The model under review builds one solid part; all positions refer to its coordinate system, in mm. Face numbers are marked on the shaded views. Coordinates: 2 decimals unless noted, no trailing zeros. Write each loop counter-clockwise with the first axis right and the second up, starting at its lowest first coordinate (ties: lowest second). Pieces come first, ordered by that corner, then holes. Notation, with made-up numbers: (67.5, 56) - (89.5, 56) arc R17 cw to (89.5, 89) - close; hole circle Ø5 at (80, -37). An arc over 180 degrees is marked (long way). Put each result on its own line as item: value.
Autodesk Inventor part; units mm, degrees
ref_plane "YZ Plane" through (0, 0, 0) normal (1, 0, 0) x (0, 1, 0)
ref_plane "XZ Plane" through (0, 0, 0) normal (0, 1, 0) x (-1, 0, 0)
ref_plane "XY Plane" through (0, 0, 0) normal (0, 0, 1) x (1, 0, 0)
sketch "Sketch2" plane through (0, 0, 0) normal (1, 0, 0) x (0, 1, 0)
  circle A0 centre (0, 0) radius 10
  circle A1 centre (0, 0) radius 12.5
  dimension "d3" = 20
  dimension "d4" = 25
extrude "Extrusion1" add sketch "Sketch2" along normal blind 15
sketch "Sketch3" plane through (0, 0, 0) normal (-1, 0, 0) x (0, 0, 1)
  circle A0 centre (0, 0) radius 10
  arc A1 (10, 0) -> (-10, 0) centre (0, 0) ccw
  circle A2 centre (0, 0) radius 12.5
  arc A3 (12.5, 0) -> (-12.5, 0) centre (0, 0) ccw
  line L0 (-12.5, 0) -> (-10, 0)
  line L1 (10, 0) -> (12.5, 0)
revolve "Revolution1" add sketch "Sketch3" angle 180 about axis through (0, 0, 10) along (0, 0, 1) picked at (-11.4487, 1.7949) contours A0 L0 A2 L1
sketch "Sketch5" plane through (15, 0, 0) normal (1, 0, 0) x (0, 0, -1)
  circle A0 centre (-8, 8) radius 1
  point P0 (0, 0)
  dimension "d9" = 2
extrude "Extrusion2" cut sketch "Sketch5" against normal blind 7
mirror "Mirror1" about plane through (0, 0, 0) normal (0, 0, 1) of "Extrusion2"
mirror "Mirror2" about plane through (0, 0, 0) normal (0, 1, 0) of "Extrusion2", "Mirror1"
properties part number "Plasmid Half 2"
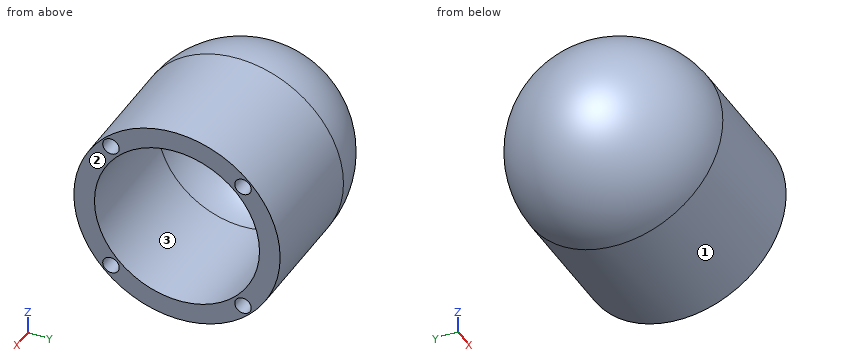
1. Consider section B-B on z = 0. State the section outline as (x, y) points, plus the area to 3 significant figures.
Determined:
outline: (0, -12.5) - (15, -12.5) - (15, -10) - (0, -10) arc R10 cw to (0, 10) - (15, 10) - (15, 12.5) - (0, 12.5) arc R12.5 ccw to start
area: 163 mm^2
2. For pin 1 Ø1.6 at (y, z) = (8, -8) entering from +X; pin 2 Ø1.6 at (y, z) = (-8, 8) entering from -X; pin 3 Ø1.5 at (y, z) = (7, -4) entering from -X, all flat-tipped, find the tip position at first contact; note any pin that passes through.
Determined:
pin 1: stops at x = 8
pin 2: stops at x = -6.76
pin 3: stops at x = -10.14
3. Consider section A-A on x = 12. State the section outline as (y, z) points.
Determined:
outline: circle Ø25 at (0, 0); hole circle Ø20 at (0, 0); hole circle Ø2 at (-8, -8); hole circle Ø2 at (-8, 8); hole circle Ø2 at (8, -8); hole circle Ø2 at (8, 8)
4. The part is to be moulded in two halves that separate along Z. For the marked faces 1, 2 and 3, say which applies: +Z half, -Z half, draft (parallel to the pull), parting line (faces both ways), or undercut.
Determined:
face 1: parting line
face 2: draft
face 3: undercut
5. Consider section D-D on x = 2. State the section outline as (y, z) points.
Determined:
outline: circle Ø25 at (0, 0); hole circle Ø20 at (0, 0)
6. To check wall thickness, follow probe 1 along Z at (x, y) = (12, -8); probe 2 along Z at (x, y) = (12, -8.5). State the ranges of each line that lie inside material, in increasing order.
Determined:
probe 1: z = -9.6 to -9, -7 to -6, 6 to 7, 9 to 9.6
probe 2: z = -9.17 to -8.87, -7.13 to -5.27, 5.27 to 7.13, 8.87 to 9.17
